```python
from build123d import *

# Parameters (mm, degrees)
SKETCH1_W                 = 1.5
SKETCH1_H                 = 45
BOSS_EXTRUDE1_DEPTH       = 16
SKETCH2_W                 = 32
SKETCH2_H                 = 10
BOSS_EXTRUDE2_DEPTH       = 16.2
M3X0_5_TAPPED_HOLE1_D     = 2.75
M3X0_5_TAPPED_HOLE1_DEPTH = 12
M3X0_5_TAPPED_HOLE1_TIP   = 0.826183351
BOSS_EXTRUDE3_DEPTH       = 5
FILLET1_R                 = 0.5
M3_CLEARANCE_HOLE1_D      = 3.4
FILLET2_R                 = 5


with BuildPart() as part:
    # Sketch1 → Boss-Extrude1 (new body, symmetric)
    with BuildSketch(Plane(origin=(0, 0, 0), x_dir=(0, 0, -1), z_dir=(1, 0, 0))):
        with Locations((0.75, 22.5)):
            Rectangle(SKETCH1_W, SKETCH1_H)
    extrude(amount=BOSS_EXTRUDE1_DEPTH, both=True)

    # Sketch2 → Boss-Extrude2 (add)
    with BuildSketch(Plane(origin=(0, 0, 0), x_dir=(1, 0, 0), z_dir=(0, 1, 0))):
        with Locations((0, -5)):
            Rectangle(SKETCH2_W, SKETCH2_H)
    extrude(amount=BOSS_EXTRUDE2_DEPTH)

    # Sketch9 → Cut-Revolve1 (revolve, cut)
    with BuildSketch(Plane(origin=(0, 0, 0), x_dir=(0, 0, -1), z_dir=(1, 0, 0))):
        Polygon((-10, 16.2), (-2, 16.2), (-2, 12), (-4, 12), (-4, 6.5), (-2, 6.5), (-2, 0), (-10, 0), align=None)
    revolve(axis=Axis((0, 0, 10), (0, 1, 0)), mode=Mode.SUBTRACT)

    # M3x0.5 Tapped Hole1
    with Locations(Plane.XY.offset(10)):
        with Locations((-11.5, 13.25), (11.5, 13.25), (-11.5, 5.25), (11.5, 5.25)):
            Hole(M3X0_5_TAPPED_HOLE1_D / 2, depth=M3X0_5_TAPPED_HOLE1_DEPTH)
            with Locations((0, 0, -(M3X0_5_TAPPED_HOLE1_DEPTH + M3X0_5_TAPPED_HOLE1_TIP / 2))):  # 118° drill point
                Cone(0, M3X0_5_TAPPED_HOLE1_D / 2, M3X0_5_TAPPED_HOLE1_TIP, mode=Mode.SUBTRACT)

    # Sketch13 → Boss-Extrude3 (add)
    with BuildSketch(Plane.XZ):
        Polygon((-7.375, -1.5), (-9.375, -3.5), (9.375, -3.5), (7.375, -1.5), align=None)
    extrude(amount=-BOSS_EXTRUDE3_DEPTH)

    # Fillet1
    fillet1_edges = [part.edges().sort_by_distance(p)[0] for p in [
        (-7.375, 2.5, -1.5),
        (7.375, 2.5, -1.5),
        (9.375, 2.5, -3.5),
        (-9.375, 2.5, -3.5),
    ]]
    fillet(fillet1_edges, radius=FILLET1_R)

    # M3 Clearance Hole1 (through all)
    with Locations(Plane.XY):
        with Locations((-10, 20.6), (-10, 40.6), (10, 40.6), (10, 20.6)):
            Hole(M3_CLEARANCE_HOLE1_D / 2)

    # Fillet2
    fillet2_edges = [part.edges().sort_by_distance(p)[0] for p in [
        (16, 45, -0.75),
        (-16, 45, -0.75),
    ]]
    fillet(fillet2_edges, radius=FILLET2_R)


solid = part.part
```
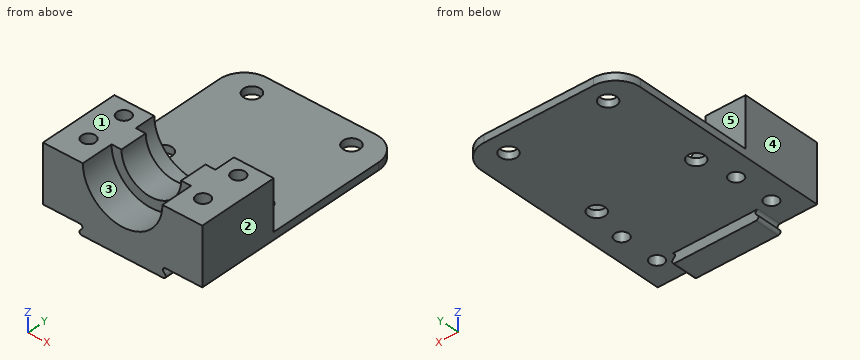
Input: part model. Units: mm. Frame: model coordinates. Face numbers are marked on the shaded views. A direction names the side the tool comes from. Give positions to 0.01 mm unless a question says otherwise; leave off trailing zeros. Order: outer loops, then holes, each group sorted by start corner. A loop starts at its lowest first (then second) coordinate and runs counter-clockwise, first axis right, second up.
1. Section C-C on x = 9.5. Return the cut outline in (y, z).
Derived:
outline: (0, -1.5) - (18.98, -1.5) - (18.98, 0) - (16.2, 0) - (16.2, 10) - (0, 10) - close; (22.22, -1.5) - (38.98, -1.5) - (38.98, 0) - (22.22, 0) - close; (42.22, -1.5) - (45, -1.5) - (45, 0) - (42.22, 0) - close
2. Section A-A on z = -1. Give the number of separate pieces and of enclosed holes in the cut face, and give its area (3 significant figures).
Derived:
separate pieces: 1
enclosed holes: 8
area: 1,370 mm2
3. Mould query, pull axis X, two halves, no side actions, for the marked faces 1, 2 and 3. Classes: released by +X, released by -X, zero draft, split by the parting line, or undercut.
Derived:
face 1: zero draft
face 2: released by +X
face 3: undercut
4. Pin query (flat end, axial travel): pin 1 (3 mm diameter, centred on x = 0.5, y = 12, fed in from +Z); pin 2 (2 mm diameter, centred on x = 4, z = -3, fed in from +Y); pin 3 (4 mm diameter, centred on x = -10, y = 20.6, fed in from +Z). Return the tip coordinate at first contact, or that it passes through.
Derived:
pin 1: stops at z = 4.34
pin 2: stops at y = 5
pin 3: stops at z = 0
5. Reachability of the marked faces 4 and 5 from +Z, -Z, +X, -X, +Y, -Y: full face, straight path, thin tool, end or side. Return the list, or none.
Derived:
face 4: +Z, -Z, -X, +Y, -Y
face 5: +Z, +X, -X, +Y
6. Material intervals for L1, parallel to Y at x = 11.5, z = 5.5 (3 decimals); L2, parallel to Y at x = -10, z = -0.65; L3, parallel to Z at x = 11.5, y = 11, sorted ascending.
Derived:
L1: y = 0 to 3.875, 6.625 to 11.875, 14.625 to 16.2
L2: y = 0 to 18.9, 22.3 to 38.9, 42.3 to 45
L3: z = -1.5 to 10
7. Section B-B on y = 13.25. Return the cut outline in (x, z) (3 decimals).
Derived:
outline: (-16, -1.5) - (-12.875, -1.5) - (-12.875, 10) - (-16, 10) - close; (-10.125, -1.5) - (10.125, -1.5) - (10.125, 10) - (8, 10) arc R8 cw to (-8, 10) - (-10.125, 10) - close; (12.875, -1.5) - (16, -1.5) - (16, 10) - (12.875, 10) - close
8. Section D-D on z = 8. Return the cut outline in (x, y) (3 decimals), and give its area (3 significant figures).
Derived:
outline: (-16, 0) - (-7.746, 0) - (-7.746, 6.5) - (-5.657, 6.5) - (-5.657, 12) - (-7.746, 12) - (-7.746, 16.2) - (-16, 16.2) - close; (5.657, 6.5) - (7.746, 6.5) - (7.746, 0) - (16, 0) - (16, 16.2) - (7.746, 16.2) - (7.746, 12) - (5.657, 12) - close; hole circle Ø2.75 at (-11.5, 5.25); hole circle Ø2.75 at (-11.5, 13.25); hole circle Ø2.75 at (11.5, 5.25); hole circle Ø2.75 at (11.5, 13.25)
area: 267 mm2
